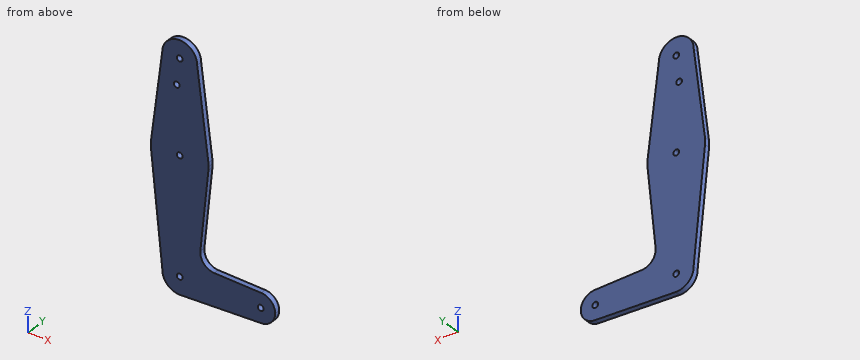
```python
from build123d import *

# Parameters (mm, degrees)
F0_R     = 1.5875
F1_DEPTH = 3.048


with BuildPart() as f1:
    # F0 (on Front) → F1 (new body)
    with BuildSketch(Plane.XZ):
        with BuildLine():
            ThreePointArc((15.750073, -1.987672), (15.843737, -0.995797), (15.875, 0))
            ThreePointArc((15.875, 0), (15.843737, 0.995797), (15.750073, 1.987672))
            ThreePointArc((15.750073, 1.987672), (0.002791, 15.875), (-15.749373, 1.99321))
            ThreePointArc((-15.749373, 1.99321), (-15.873827, 0.192943), (-15.793167, -1.609816))
            ThreePointArc((-15.793167, -1.609816), (-0.190153, -15.873861), (15.750073, -1.987672))
        make_face()
        Circle(F0_R, mode=Mode.SUBTRACT)
        with BuildLine():
            ThreePointArc((-15.749373, 1.99321), (0.002791, 15.875), (15.750073, 1.987672))
            Line((15.750073, 1.987672), (9.589916, 50.8))
            ThreePointArc((9.589916, 50.8), (0.065367, 41.210307), (-9.589025, 50.66927))
            Line((-9.589025, 50.66927), (-15.749373, 1.99321))
        make_face()
        with Locations((-1.5875, 36.490685)):
            Circle(F0_R, mode=Mode.SUBTRACT)
        with BuildLine():
            Line((11.339253, -45.910697), (15.750073, -1.987672))
            ThreePointArc((15.750073, -1.987672), (-0.190153, -15.873861), (-15.793167, -1.609816))
            Line((-15.793167, -1.609816), (-9.519021, -63.16257))
            ThreePointArc((-9.519021, -63.16257), (0.168741, -53.976495), (9.525, -63.5))
            ThreePointArc((9.525, -63.5), (6.970557, -69.991299), (0.677344, -73.000886))
            Line((0.677344, -73.000886), (44.732405, -71.432475))
            ThreePointArc((44.732405, -71.432475), (36.5125, -63.5), (44.732405, -55.567525))
            Line((44.732405, -55.567525), (18.966809, -54.65024))
            ThreePointArc((18.966809, -54.65024), (13.259898, -51.932727), (11.339253, -45.910697))
        make_face()
        with BuildLine():
            ThreePointArc((-9.589025, 50.66927), (0.065367, 41.210307), (9.589916, 50.8))
            ThreePointArc((9.589916, 50.8), (-0.065367, 60.389693), (-9.589025, 50.66927))
        make_face()
        with Locations((0, 50.8)):
            Circle(F0_R, mode=Mode.SUBTRACT)
        with BuildLine():
            ThreePointArc((9.525, -63.5), (0.168741, -53.976495), (-9.519021, -63.16257))
            ThreePointArc((-9.519021, -63.16257), (-6.853453, -70.114817), (0, -73.025))
            Line((0, -73.025), (0.677344, -73.000886))
            ThreePointArc((0.677344, -73.000886), (6.970557, -69.991299), (9.525, -63.5))
        make_face()
        with Locations((0, -63.5)):
            Circle(F0_R, mode=Mode.SUBTRACT)
        with BuildLine():
            Line((0.677344, -73.000886), (0, -73.025))
            ThreePointArc((0, -73.025), (0.338886, -73.01897), (0.677344, -73.000886))
        make_face()
        with BuildLine():
            ThreePointArc((52.3875, -63.5), (50.161633, -57.98809), (44.732405, -55.567525))
            ThreePointArc((44.732405, -55.567525), (36.5125, -63.5), (44.732405, -71.432475))
            ThreePointArc((44.732405, -71.432475), (50.161633, -69.01191), (52.3875, -63.5))
        make_face()
        with Locations((44.45, -63.5)):
            Circle(F0_R, mode=Mode.SUBTRACT)
    extrude(amount=F1_DEPTH)


solid = f1.part
```
Model file for the job. Use its own axes, mm. Coordinates: 2 decimals unless noted, no trailing zeros. Order: outer loops, then holes, each group sorted by start corner. A loop starts at its lowest first (then second) coordinate and runs counter-clockwise, first axis right, second up. Notation, with made-up numbers: (54.25, 48.5) -> (96.25, 48.5) arc R23 ccw to (96.25, 70.5) -> close; hole circle Ø2 at (29.25, 79.5). An arc over 180 degrees is marked (long way). Return JSON: item names as keys, results as strings.
Item 1: Pin check, flat tip, straight feed: P1, Ø3, axis at x = 0, z = 0, coming from the +Y side. Stop position of the tip, or through.
Model answer:
{"P1": "passes through"}
Item 2: Wall check: line 1 along Z through (x, y) = (36, -2.2); line 2 along X through (y, z) = (-0.6, 9); line 3 along X through (y, z) = (-2.55, -9). Give the ranges that are in metal, low to high. Write a range as from..to.
Model answer:
{"line 1": "z = -71.74..-55.26", "line 2": "x = -14.86..14.87", "line 3": "x = -15.04..15.05"}
Item 3: Slice it at A-A (y = -2.1). Count the separate pieces of the cut face and the enclosed holes in it, then the cut area to 3 significant figures.
Model answer:
{"separate pieces": "1", "enclosed holes": "5", "area": "3,890 mm²"}
Item 4: Slice it at B-B (z = -14). Write the cut outline in (x, y), then the cut area to 3 significant figures.
Model answer:
{"outline": "(-14.53, -3.05) -> (14.54, -3.05) -> (14.54, 0) -> (-14.53, 0) -> close", "area": "88.6 mm²"}
Item 5: Slice it at C-C (x = 7). Write the cut outline in (y, z), then the cut area to 3 significant figures.
Model answer:
{"outline": "(-3.05, -72.78) -> (0, -72.78) -> (0, 57.35) -> (-3.05, 57.35) -> close", "area": "397 mm²"}
